from build123d import *

# Parameters (mm, degrees)
BOSS_EXTRUDE1_DEPTH = 21.6
SKETCH2_OUTSIDE_W   = 131.808
SKETCH2_OUTSIDE_H   = 138.238
SKETCH2_OUTSIDE_R   = 20.667093795
CUT_EXTRUDE2_DEPTH  = 21.6
CUT_EXTRUDE2_DRAFT  = -60
M24_TAPPED_HOLE1_D  = 21


with BuildPart() as part:
    # Sketch1 → Boss-Extrude1 (new body)
    with BuildSketch(Plane(origin=(0, 0, 0), x_dir=(0, 0, -1), z_dir=(1, 0, 0))):
        Polygon((0, -24), (20.784609691, -12), (20.784609691, 12), (0, 24), (-20.784609691, 12), (-20.784609691, -12), align=None)
    extrude(amount=BOSS_EXTRUDE1_DEPTH)


with BuildPart() as cut_extrude2_tool:
    # Sketch2 outside → Cut-Extrude2 (with draft: the straight prism first)
    with BuildSketch(Plane(origin=(21.6, 0, 0), x_dir=(0, 0, -1), z_dir=(1, 0, 0))):
        Rectangle(SKETCH2_OUTSIDE_W, SKETCH2_OUTSIDE_H)
        Circle(SKETCH2_OUTSIDE_R, mode=Mode.SUBTRACT)
    extrude(amount=-CUT_EXTRUDE2_DEPTH)
    # Cut-Extrude2: the draft: its side faces are tilted about the plane it starts from
    cut_extrude2_sides = [cut_extrude2_tool.faces().sort_by_distance(p)[0] for p in [
        (10.8, -69.119, 0),
        (10.8, 0, -65.904),
        (10.8, 69.119, 0),
        (10.8, 0, 65.904),
        (10.8, 0, 20.667093795),
    ]]
    draft(cut_extrude2_sides, Plane(origin=(21.6, 0, 0), x_dir=(0, 0, -1), z_dir=(1, 0, 0)), CUT_EXTRUDE2_DRAFT)


with BuildPart() as part_1:
    add(part.part)

    # Cut-Extrude2: cut by cut_extrude2_tool
    add(cut_extrude2_tool.part, mode=Mode.SUBTRACT)

    # M24 Tapped Hole1 (through all)
    with Locations(Plane(origin=(21.6, 0, 0), x_dir=(0, 0, -1), z_dir=(1, 0, 0))):
        with Locations((0, 0)):
            Hole(M24_TAPPED_HOLE1_D / 2)


solid = part_1.part
CAD build for the part. Positions are in the model's coordinates, mm. Round coordinates to 2 decimals unless told otherwise and drop trailing zeros. Write each loop counter-clockwise with the first axis right and the second up, starting at its lowest first coordinate (ties: lowest second). Pieces come first, ordered by that corner, then holes. Notation, with made-up numbers: (-32.75, 52) -> (-19.75, 52) arc R21 cw to (-19.75, 67) -> close; hole circle Ø10 at (52, 77.5). An arc over 180 degrees is marked (long way). Answer as a JSON object with one key per item and string values.
(1) Pin check, flat tips, straight feed: P1, Ø12.5, axis at y = 0, z = 0, coming from the +X side; P2, Ø12, axis at x = 15.5, z = -9, coming from the +Y side; P3, Ø5, axis at x = 3, z = 11, coming from the -Y side; P4, Ø5, axis at x = 14.5, z = 16, coming from the +Y side. Stop position of each tip, or through.
Reported:
{"P1": "passes through", "P2": "stops at y = 22.27", "P3": "stops at y = -19.09", "P4": "stops at y = 16.21"}
(2) Two-plate mould, pull along Z, no slides. Class faces 1 (the face through (21.5, 6.8, -19.7)), 2 (the face through (10.6, 3.2, 10)), 3 (the face through (0, -5, 10)): +Z half, -Z half, draft (parallel to the pull), parting line (faces both ways), or undercut.
Reported:
{"face 1": "parting line", "face 2": "undercut", "face 3": "draft"}
(3) Band-saw the part on A-A, the plane x = 8. List the corners of the cut face in (y, z), then the cut area to 3 significant figures.
Reported:
{"outline": "(-24, 0) -> (-12, -20.78) -> (12, -20.78) -> (24, 0) -> (12, 20.78) -> (-12, 20.78) -> close; hole circle Ø21 at (0, 0)", "area": "1,150 mm^2"}
(4) Probe probe 1 along Y at (x, z) = (12.75, 0); probe 2 along Z at (x, y) = (12.75, -6.5); probe 3 along Y at (x, z) = (19.25, 2). List the from-to ranges inside material, lowest first. Write a range as [from, to].
Reported:
{"probe 1": "y = [-24, -10.5], [10.5, 24]", "probe 2": "z = [-20.78, -8.25], [8.25, 20.78]", "probe 3": "y = [-22.85, -10.31], [10.31, 22.85]"}
(5) Band-saw the part on B-B, the plane y = 0. List the corners of the cut face in (x, z).
Reported:
{"outline": "(0, -20.78) -> (21.53, -20.78) -> (21.6, -20.67) -> (21.6, -10.5) -> (0, -10.5) -> close; (0, 10.5) -> (21.6, 10.5) -> (21.6, 20.67) -> (21.53, 20.78) -> (0, 20.78) -> close"}
